Drawing for the job (mm, zero at the part's lowest x, y, z). A direction names the side the tool comes from. Round coordinates to 2 decimals unless told otherwise and drop trailing zeros. Order: outer loops, then holes, each group sorted by start corner. A loop starts at its lowest first (then second) coordinate and runs counter-clockwise, first axis right, second up. Notation, with made-up numbers: M 35.5,-17.75 L 42.5,-17.75 A12 cw 42.5,4.25 Z; hole C 62.5,72.5 d8. An arc over 180 degrees is marked long. One line per item, written item: value. Start each with the question number.
Item 1: Band-saw the part on B-B, the plane y = 19. Write the cut outline in (x, z) (3 decimals), then the cut area to 3 significant figures.
Item 2: Tool access for the marked faces 1 and 2: list every direction of +Z, -Z, +X, -X, +Y, -Y with a clear straight run to the whole face (end or side of a thin tool).
Item 3: Two-plate mould, pull along Z, no slides. Class the marked faces 3, 4 and 5: +Z half, -Z half, draft (parallel to the pull), parting line (faces both ways), or undercut.
Item 4: Probe L1, parallel to Y at x = 129, z = 82; L2, parallel to X at y = 6.5, z = 72 (1 decimal); L3, parallel to Y at x = 41, z = 48.5. List the from-to ranges inside material, lowest first.
Item 5: Pin check, flat tips, straight feed: pin 1 (12 mm diameter, centred on x = 16, z = 76.67, fed in from +Y); pin 2 (24 mm diameter, centred on x = 121.075, z = 16, fed in from +Y); pin 3 (1.5 mm diameter, centred on y = 54.5, z = 41.5, fed in from -X) (1 decimal); pin 4 (4 mm diameter, centred on x = 51.5, z = 106.5, fed in from +Y). Stop position of each tip, or through.
Item 6: Band-saw the part on C-C, the plane y = 57.5. Write the cut outline in (x, z) (3 decimals).
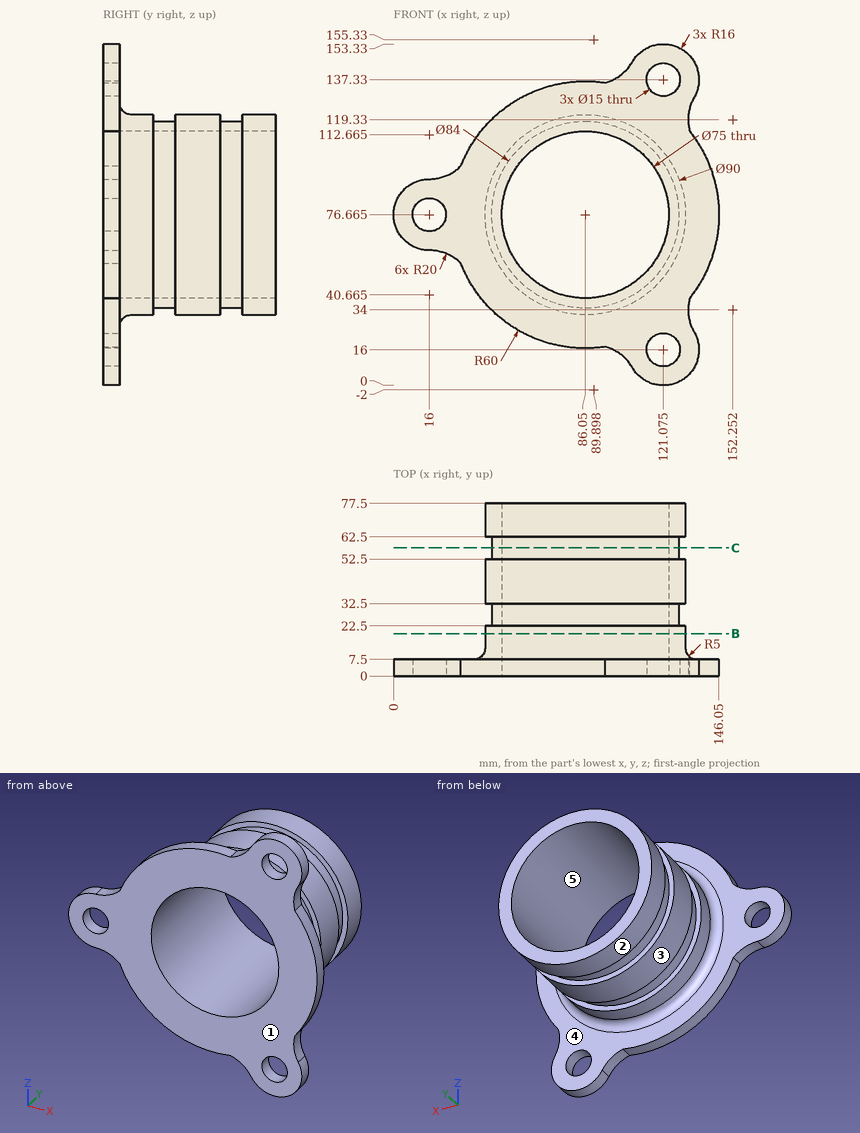
Output:
1. outline: C 86.05,76.665 d90; hole C 86.05,76.665 d75
1. area: 1,940 mm²
2. face 1: +Z, -Z, +X, -X, -Y
2. face 2: +Y
3. face 3: parting line
3. face 4: draft
3. face 5: undercut
4. L1: y = 0 to 22.5, 32.5 to 52.5, 62.5 to 77.5
4. L2: x = 0.7 to 10.1, 21.9 to 48.8, 123.3 to 145.9
4. L3: y = 0 to 7.5
5. pin 1: passes through
5. pin 2: stops at y = 7.5
5. pin 3: stops at x = 62
5. pin 4: stops at y = 77.5
6. outline: C 86.05,76.665 d84; hole C 86.05,76.665 d75
